Read the model definition and answer for the solid it produces. Units are mm, in the model's axes. A direction names the side the tool comes from. Round coordinates to 2 decimals unless told otherwise and drop trailing zeros. Loops run counter-clockwise (first coordinate to the right, second up) from the corner with the lowest first, then second, coordinate; pieces in that order, holes last. Notation, with made-up numbers: (-31.5, 69.25) -> (-0.5, 69.25) arc R19 cw to (-0.5, 74.25) -> close; hole circle Ø2 at (82, 52). An arc over 180 degrees is marked (long way). Put each result on its own line as item: value.
from build123d import *

# Parameters (mm, degrees)
CROQUIS1_W              = 20
CROQUIS1_H              = 20
SALIENTE_EXTRUIR1_DEPTH = 150
CROQUIS2_R              = 2.5
CORTAR_EXTRUIR1_DEPTH   = 151.665191733
CROQUIS3_R              = 4
CORTAR_EXTRUIR2_DEPTH   = 152.657508881


with BuildPart() as part:
    # Croquis1 → Saliente-Extruir1 (new, symmetric)
    with BuildSketch(Plane.XY):
        Rectangle(CROQUIS1_W, CROQUIS1_H)
    extrude(amount=SALIENTE_EXTRUIR1_DEPTH, both=True)

    # Croquis2 → Cortar-Extruir1 (cut, through all)
    with BuildSketch(Plane(origin=(0, 0, 0), x_dir=(0, 0, -1), z_dir=(1, 0, 0))):
        Circle(CROQUIS2_R)
        with Locations((140, 0)):
            Circle(CROQUIS2_R)
        with Locations(Location((-140, 0, 0), (0, 0, 180))):
            Circle(CROQUIS2_R)
    extrude(amount=-CORTAR_EXTRUIR1_DEPTH, mode=Mode.SUBTRACT)

    # Croquis3 → Cortar-Extruir2 (cut, through all)
    with BuildSketch(Plane.ZY.offset(10)):
        with Locations((80, 0)):
            Circle(CROQUIS3_R)
        with Locations(Location((-80, 0, 0), (0, 0, 180))):
            Circle(CROQUIS3_R)
    extrude(amount=-CORTAR_EXTRUIR2_DEPTH, mode=Mode.SUBTRACT)


solid = part.part
Item 1: The part is cut by section A-A (y = 0). Determine the outline of the cut face in (x, z), then the cut area to 3 significant figures.
Derived:
outline: (-10, -150) -> (10, -150) -> (10, -84) -> (-10, -84) -> (-10, -137.5) -> (0, -137.5) -> (0, -142.5) -> (-10, -142.5) -> close; (-10, -76) -> (10, -76) -> (10, 76) -> (-10, 76) -> (-10, 2.5) -> (0, 2.5) -> (0, -2.5) -> (-10, -2.5) -> close; (-10, 84) -> (10, 84) -> (10, 150) -> (-10, 150) -> (-10, 142.5) -> (0, 142.5) -> (0, 137.5) -> (-10, 137.5) -> close
area: 5,530 mm^2
Item 2: A flat-ended cylindrical pin translates along its axis: pin 1 Ø1.5 at (y, z) = (1, 0.5) entering from -X. Find the tip coordinate at first contact, or state that the pin passes through.
Derived:
pin 1: stops at x = 0
Item 3: For a pull along Z with two mould halves and no side action, classify faces 1 (the flat face through (-10, 2, 2)), 2 (the cylindrical face through (-4.93, -0.751, 142.385)), 3 (the cylindrical face through (0, 0, 76)), 4 (the flat face through (0, 0, -150)) as pulls with the +Z half, pulls with the -Z half, needs draft (parallel to the pull), parting line crosses it, or undercut.
Derived:
face 1: needs draft
face 2: undercut
face 3: undercut
face 4: pulls with the -Z half
Item 4: Find the intervals of material crossed by line 1 along Z through (x, y) = (-5.75, -0.5); line 2 along Z through (x, y) = (5.5, -0.5); line 3 along Y through (x, z) = (-1, -80), in increasing order.
Derived:
line 1: z = -150 to -142.45, -137.55 to -83.97, -76.03 to -2.45, 2.45 to 76.03, 83.97 to 137.55, 142.45 to 150
line 2: z = -150 to -83.97, -76.03 to 76.03, 83.97 to 150
line 3: y = -10 to -4, 4 to 10
Item 5: The part is cut by section D-D (z = 0). Determine the outline of the cut face in (x, y).
Derived:
outline: (-10, -10) -> (10, -10) -> (10, 10) -> (-10, 10) -> (-10, 2.5) -> (0, 2.5) -> (0, -2.5) -> (-10, -2.5) -> close
Item 6: Which of the six approach directions +Z, -Z, +X, -X, +Y, -Y give full straight-line access (tool end or side, diameter ignored) to faces 5 (the flat face through (0, 0, 140)), 6 (the cylindrical face through (0, 0, -76))?
Derived:
face 5: -X
face 6: +X, -X
Item 7: The part is cut by section B-B (z = -80). Determine the outline of the cut face in (x, y).
Derived:
outline: (-10, -10) -> (10, -10) -> (10, -4) -> (-10, -4) -> close; (-10, 4) -> (10, 4) -> (10, 10) -> (-10, 10) -> close
Item 8: The part is cut by section C-C (x = -6.5). Determine the outline of the cut face in (y, z).
Derived:
outline: (-10, -150) -> (10, -150) -> (10, 150) -> (-10, 150) -> close; hole circle Ø8 at (0, -80); hole circle Ø8 at (0, 80); hole circle Ø5 at (0, -140); hole circle Ø5 at (0, 0); hole circle Ø5 at (0, 140)
